Check sheet for the modelled part. Datum: model origin and axes. Units: mm. A direction names the side the tool comes from. Give positions to 0.01 mm unless a question says otherwise; leave off trailing zeros. Write each loop counter-clockwise with the first axis right and the second up, starting at its lowest first coordinate (ties: lowest second). Pieces come first, ordered by that corner, then holes.
from build123d import *

# Parameters (mm, degrees)
SKETCH1_R               = 22.21
SKETCH1_R_2             = 19.91
BOSS_EXTRUDE1_DEPTH     = 146.05
CUT_EXTRUDE2_REACH      = 157.431
CUT_EXTRUDE2_END_RADIUS = 19.91
SKETCH5_R               = 14.8463
CUT_EXTRUDE3_REACH      = 156.263
SKETCH4_R               = 9.0424


with BuildPart() as part:
    # Sketch1 → Boss-Extrude1 (new body)
    with BuildSketch(Plane.XY):
        with Locations((-0.049436733, 0)):
            Circle(SKETCH1_R)
        with Locations((-0.049436733, 0)):
            Circle(SKETCH1_R_2, mode=Mode.SUBTRACT)
    extrude(amount=BOSS_EXTRUDE1_DEPTH)

    # Cut-Extrude2: up to this cylinder (the profile starts outside it)
    cut_extrude2_end = Plane(origin=(-0.049436733, 0, 127.35), z_dir=(0, 0, -1)) * Cylinder(CUT_EXTRUDE2_END_RADIUS, 355.682, mode=Mode.PRIVATE)
    # Sketch5 → Cut-Extrude2 (cut, up to the surface)
    with BuildSketch(Plane(origin=(11.092620184, -19.212981748, 146.05), x_dir=(-0.8650599616540103, -0.5016684789212517, 0), z_dir=(0.5016684789212515, -0.8650599616540102, 0)), mode=Mode.PRIVATE) as cut_extrude2_sk1:
        with Locations(Location((-0.049436639, 18.7, 0), (0, 0, 180))):
            Circle(SKETCH5_R)
    cut_extrude2_tool1 = extrude(cut_extrude2_sk1.sketch, amount=-CUT_EXTRUDE2_REACH, mode=Mode.PRIVATE) - cut_extrude2_end
    add(cut_extrude2_tool1.solids().sort_by_distance((11.135386, -19.188181, 127.35))[0], mode=Mode.SUBTRACT)

    # Sketch4 → Cut-Extrude3 (cut, up to next)
    with BuildSketch(Plane(origin=(22.160563267, 0, 146.05), x_dir=(0, 0, -1), z_dir=(1, 0, 0)), mode=Mode.PRIVATE) as cut_extrude3_sk1:
        with Locations(Location((126.05, 10.153466667, 0), (0, 0, 90))):
            Circle(SKETCH4_R)
    cut_extrude3_tool1 = extrude(cut_extrude3_sk1.sketch, amount=-CUT_EXTRUDE3_REACH, mode=Mode.PRIVATE) & part.part
    add(cut_extrude3_tool1.solids().sort_by_distance((22.160563, 10.153467, 20))[0], mode=Mode.SUBTRACT)


solid = part.part
1) Sectioned sample at C-C on z = 99. Record the boundary of the cut face in (x, y).
2) Access from +Z, -Z, +X, -X, +Y, -Y to the whole of each face (thin tool, end or side, straight path). Record for faces 1 (the cylindrical face through (13.098, 17.635, 14.921)), 2 (the cylindrical face through (-19.94, 0.88, 72)).
3) Sectioned sample at B-B on x = -18. Record the boundary of the cut face in (y, z), then the cut area to 3 significant figures.
4) Scan lines: L1, parallel to Y at x = -0.5, z = 82; L2, parallel to Z at x = 12, y = -16.5; L3, parallel to Y at x = 12.5, z = 85.5. Record each from-to range of solid material in increasing order.
5) Draft check along X on faces 3 (the cylindrical face through (19.55, -8.74, 135.33)), 4 (the cylindrical face through (-16.42, 15.01, 72)), 5 (the flat face through (-3, 20, 146.05)). Enter one of: +X half, -X half, draft (parallel to the pull), parting line (faces both ways), or undercut.
6) Sectioned sample at A-A on y = -1.5. Record the boundary of the cut face in (x, z), then the cut area to 3 significant figures.
7) Sectioned sample at D-D on x = 14.5. Give the number of separate pieces and of enclosed holes in the cut face, then the cut area to 3 significant figures.
8) Gauge pin test, flat ends, axial feed: pin 1 (21 mm diameter, centred on y = 10.15, z = 20, fed in from -X); pin 2 (8 mm diameter, centred on x = -9.5, z = 48, fed in from +Y); pin 3 (1 mm diameter, centred on y = 16.5, z = 15.5, fed in from -X). Record the tip position at first contact, or that the pin passes through.
Answers below:
1. outline: circle Ø44.42 at (-0.05, 0); hole circle Ø39.82 at (-0.05, 0)
2. face 1: +X
2. face 2: +Z, -Z
3. outline: (-13.08, 0) - (-8.61, 0) - (-8.61, 146.05) - (-13.08, 146.05) - close; (8.61, 0) - (13.08, 0) - (13.08, 146.05) - (8.61, 146.05) - close
3. area: 1,300 mm2
4. L1: y = -22.21 to -19.9, 19.9 to 22.21
4. L2: z = 0 to 112.65, 142.05 to 146.05
4. L3: y = -18.32 to -15.46, 15.46 to 18.32
5. face 3: undercut
5. face 4: parting line
5. face 5: draft
6. outline: (-22.21, 0) - (-19.9, 0) - (-19.9, 146.05) - (-22.21, 146.05) - close; (19.8, 0) - (22.11, 0) - (22.11, 146.05) - (19.8, 146.05) - close
6. area: 674 mm2
7. separate pieces: 4
7. enclosed holes: 0
7. area: 795 mm2
8. pin 1: stops at x = -22.26
8. pin 2: stops at y = 21.53
8. pin 3: stops at x = -15.45
